```python
from build123d import *

# Parameters (mm, degrees)
SKETCH1_R           = 2.3495
SKETCH1_R_2         = 2.54
BOSS_EXTRUDE1_DEPTH = 1.6002


with BuildPart() as part:
    # Sketch1 → Boss-Extrude1 (new body)
    with BuildSketch(Plane.XY):
        with BuildLine():
            Line((0, 0), (0, 15.24))
            Line((0, 15.24), (66.713584346, 52.060343069))
            Line((66.713584346, 52.060343069), (121.323584346, 52.482745441))
            ThreePointArc((121.323584346, 52.482745441), (126.52255489, 45.138126941), (124.63483314, 36.339875852))
            Line((124.63483314, 36.339875852), (63.5, 0))
            Line((63.5, 0), (0, 0))
        make_face()
        with Locations((10.16, 9.525)):
            Circle(SKETCH1_R, mode=Mode.SUBTRACT)
        with Locations((50.8, 9.525)):
            Circle(SKETCH1_R, mode=Mode.SUBTRACT)
        with Locations((118.841606936, 42.303243693)):
            Circle(SKETCH1_R_2, mode=Mode.SUBTRACT)
    extrude(amount=-BOSS_EXTRUDE1_DEPTH)


solid = part.part
```
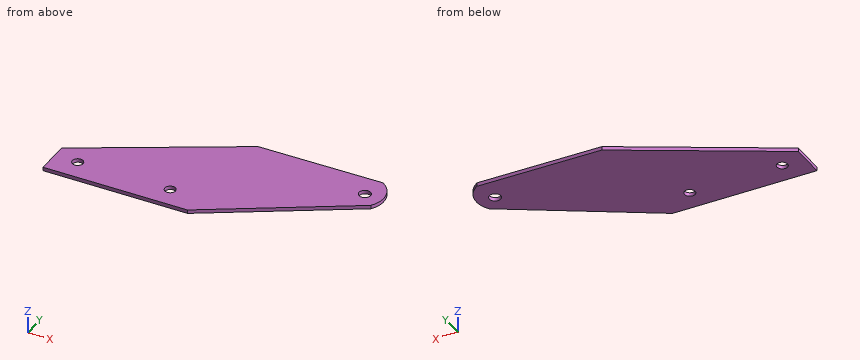
Work out the finished part from the listing and answer in its coordinate system (mm). Give positions to 0.01 mm unless a question says otherwise; leave off trailing zeros. Order: outer loops, then holes, each group sorted by start corner. A loop starts at its lowest first (then second) coordinate and runs counter-clockwise, first axis right, second up.
1. Section C-C, the plane x = 10.16 is taken. Determine the outline of the cut face in (y, z).
Result sheet:
outline: (0, -1.6) - (7.18, -1.6) - (7.18, 0) - (0, 0) - close; (11.87, -1.6) - (20.85, -1.6) - (20.85, 0) - (11.87, 0) - close
2. This flat-tipped pin is pushed along its axis until it touches: P1, Ø4, axis at x = 50.8, y = 9.525, coming from the -Z side. Where does it stop, or does it pass through?
Result sheet:
P1: passes through
3. Section D-D, the plane y = 46.5 is taken. Determine the outline of the cut face in (x, z), and give its area (3 significant figures).
Result sheet:
outline: (56.64, -1.6) - (126.15, -1.6) - (126.15, 0) - (56.64, 0) - close
area: 111 mm2
4. Section A-A, the plane x = 52 is taken. Determine the outline of the cut face in (y, z).
Result sheet:
outline: (0, -1.6) - (7.51, -1.6) - (7.51, 0) - (0, 0) - close; (11.54, -1.6) - (43.94, -1.6) - (43.94, 0) - (11.54, 0) - close
5. Straight lines are drawn through the part: L1, parallel to X at y = 9, z = -0.25; L2, parallel to X at y = 8, z = -0.05; L3, parallel to X at y = 43, z = -0.25. For each, find the intervals that lie inside material, in ascending order.
Result sheet:
L1: x = 0 to 7.87, 12.45 to 48.51, 53.09 to 78.64
L2: x = 0 to 8.37, 11.95 to 49.01, 52.59 to 76.96
L3: x = 50.3 to 116.4, 121.28 to 126.75
6. Section B-B, the plane z = -1.05 is taken. Determine the outline of the cut face in (x, y) (1 decimal), and give its area (3 significant figures).
Result sheet:
outline: (0, 0) - (63.5, 0) - (124.6, 36.3) arc R11.2 ccw to (121.3, 52.5) - (66.7, 52.1) - (0, 15.2) - close; hole circle Ø4.7 at (10.2, 9.5); hole circle Ø4.7 at (50.8, 9.5); hole circle Ø5.1 at (118.8, 42.3)
area: 4,120 mm2
